Work out the finished part from the listing and answer in its coordinate system (mm). A direction names the side the tool comes from. Round coordinates to 2 decimals unless told otherwise and drop trailing zeros. Loops run counter-clockwise (first coordinate to the right, second up) from the corner with the lowest first, then second, coordinate; pieces in that order, holes last. Notation, with made-up numbers: (85, 84.25) - (101, 84.25) arc R24 cw to (101, 117.25) - close; hole circle Ø2 at (-37, 3.5). An arc over 180 degrees is marked (long way). Answer as CSV lines item,"result". Start each with the question number.
Q1. The mould has two halves that part along X. Classify faces 5 (the face through (1, 10, 10.16)), 6 (the face through (-10.39, 10.36, 6.26)), 7 (the face through (35, 8, 13.97)): +X half, -X half, draft (parallel to the pull), parting line (faces both ways), or undercut.
Q2. Straight lines are drawn through the part: L1, parallel to X at y = -0.75, z = 2; L2, parallel to X at y = 4.5, z = 10.25; L3, parallel to Y at x = -5.5, z = 12.5. For each, find the intervals that lie inside material, in ascending order. Write a range as [from, to].
Q3. Section D-D on z = 2.25 is taken. Count the separate pieces of the cut face and the enclosed holes in it, then the cut area to 3 significant figures.
Q4. Section A-A on y = -5 is taken. Write down the section's boundary in (x, z) (1 decimal), then the cut area to 3 significant figures.
Q5. For faces 1 (the face through (38.5, -7.43, 13.59)), 2 (the face through (20.7, 8.13, 13.61)), 3 (the face through (-5, -7, 10.16)), 4 (the face through (-7.97, 4.65, 13.61)), determine the directions among +Z, -Z, +X, -X, +Y, -Y from which every point of the face is accessible in a straight line to the end or side of a thin tool.
Q6. Section C-C on y = 2.25 is taken. Write down the section's boundary in (x, z) (1 decimal), then the cut area to 3 significant figures.
Q7. Section B-B on x = 26.5 is taken. Write down the section's boundary in (y, z).
Q8. Each of these flat-tipped pins is pushed along its axis until it touches: pin 1 Ø2 at (x, z) = (36.5, 11.5) entering from -Y; pin 2 Ø2 at (x, y) = (28, -7.5) entering from -Z; pin 3 Ø1.5 at (x, y) = (0, -11.5) entering from +Z; pin 4 Ø8 at (y, z) = (-9.5, 8) entering from -X. Where does it stop, or does it pass through?
```python
from build123d import *

# Parameters (mm, degrees)
F1_DEPTH        = 10.16
F2_DEPTH        = 13.97
F3_DEPTH        = 10.16
F8_R            = 5.08
F9_R            = 1.27
F11_D           = 4.445
F11_CSINK_D     = 8.89
F11_CSINK_ANGLE = 90


with BuildPart() as f1:
    # F0 (on Top) → F1 (new body)
    with BuildSketch(Plane.XY):
        with BuildLine():
            Line((-4.2164, 11.888180349), (-11.8364, 11.888180349))
            Line((-11.8364, 11.888180349), (-11.8364, 4.268180349))
            Line((-11.8364, 4.268180349), (-6.8157005053, 4.268180349))
            ThreePointArc((-6.8157005053, 4.268180349), (-5.6470856878, 5.6988660368), (-4.2164, 6.8674808543))
            Line((-4.2164, 6.8674808543), (-4.2164, 11.888180349))
        make_face()
        with BuildLine():
            Line((-4.2164, 4.268180349), (-4.2164, 6.8674808543))
            ThreePointArc((-4.2164, 6.8674808543), (-5.6470856878, 5.6988660368), (-6.8157005053, 4.268180349))
            Line((-6.8157005053, 4.268180349), (-4.2164, 4.268180349))
        make_face()
        with BuildLine():
            Line((13.5636, 11.888180349), (5.9436, 11.888180349))
            Line((5.9436, 11.888180349), (5.9436, 6.8674808543))
            ThreePointArc((5.9436, 6.8674808543), (7.3742856878, 5.6988660368), (8.5429005053, 4.268180349))
            Line((8.5429005053, 4.268180349), (13.5636, 4.268180349))
            Line((13.5636, 4.268180349), (13.5636, 11.888180349))
        make_face()
        with BuildLine():
            Line((13.5636, -13.511819651), (13.5636, -5.891819651))
            Line((13.5636, -5.891819651), (8.5429005053, -5.891819651))
            ThreePointArc((8.5429005053, -5.891819651), (7.3742856878, -7.3225053388), (5.9436, -8.4911201562))
            Line((5.9436, -8.4911201562), (5.9436, -13.511819651))
            Line((5.9436, -13.511819651), (13.5636, -13.511819651))
        make_face()
        with BuildLine():
            Line((-4.2164, -8.4911201562), (-4.2164, -13.511819651))
            Line((-4.2164, -13.511819651), (5.9436, -13.511819651))
            Line((5.9436, -13.511819651), (5.9436, -8.4911201562))
            ThreePointArc((5.9436, -8.4911201562), (0.8636, -10.019319651), (-4.2164, -8.4911201562))
        make_face()
        with BuildLine():
            Line((-6.8157005053, -5.891819651), (-11.8364, -5.891819651))
            Line((-11.8364, -5.891819651), (-11.8364, -13.511819651))
            Line((-11.8364, -13.511819651), (-4.2164, -13.511819651))
            Line((-4.2164, -13.511819651), (-4.2164, -8.4911201562))
            ThreePointArc((-4.2164, -8.4911201562), (-5.6470856878, -7.3225053388), (-6.8157005053, -5.891819651))
        make_face()
        with BuildLine():
            Line((-6.8157005053, 4.268180349), (-11.8364, 4.268180349))
            Line((-11.8364, 4.268180349), (-11.8364, -5.891819651))
            Line((-11.8364, -5.891819651), (-6.8157005053, -5.891819651))
            ThreePointArc((-6.8157005053, -5.891819651), (-8.3439, -0.811819651), (-6.8157005053, 4.268180349))
        make_face()
        with BuildLine():
            Line((13.5636, -5.891819651), (13.5636, 4.268180349))
            Line((13.5636, 4.268180349), (8.5429005053, 4.268180349))
            ThreePointArc((8.5429005053, 4.268180349), (9.6807768626, 1.8406223227), (10.0711, -0.811819651))
            ThreePointArc((10.0711, -0.811819651), (9.6807768626, -3.4642616247), (8.5429005053, -5.891819651))
            Line((8.5429005053, -5.891819651), (13.5636, -5.891819651))
        make_face()
        with BuildLine():
            Line((5.9436, 11.888180349), (-4.2164, 11.888180349))
            Line((-4.2164, 11.888180349), (-4.2164, 6.8674808543))
            ThreePointArc((-4.2164, 6.8674808543), (0.8636, 8.395680349), (5.9436, 6.8674808543))
            Line((5.9436, 6.8674808543), (5.9436, 11.888180349))
        make_face()
        with BuildLine():
            ThreePointArc((8.5429005053, 4.268180349), (7.3742856878, 5.6988660368), (5.9436, 6.8674808543))
            Line((5.9436, 6.8674808543), (5.9436, 4.268180349))
            Line((5.9436, 4.268180349), (8.5429005053, 4.268180349))
        make_face()
        with BuildLine():
            Line((5.9436, -5.891819651), (5.9436, -8.4911201562))
            ThreePointArc((5.9436, -8.4911201562), (7.3742856878, -7.3225053388), (8.5429005053, -5.891819651))
            Line((8.5429005053, -5.891819651), (5.9436, -5.891819651))
        make_face()
        with BuildLine():
            Line((-4.2164, -5.891819651), (-6.8157005053, -5.891819651))
            ThreePointArc((-6.8157005053, -5.891819651), (-5.6470856878, -7.3225053388), (-4.2164, -8.4911201562))
            Line((-4.2164, -8.4911201562), (-4.2164, -5.891819651))
        make_face()
    extrude(amount=F1_DEPTH)

    # F0 (on Top) → F2 (join)
    with BuildSketch(Plane.XY):
        with BuildLine():
            Line((-6.8157005053, -5.891819651), (-11.8364, -5.891819651))
            Line((-11.8364, -5.891819651), (-11.8364, -13.511819651))
            Line((-11.8364, -13.511819651), (-4.2164, -13.511819651))
            Line((-4.2164, -13.511819651), (-4.2164, -8.4911201562))
            ThreePointArc((-4.2164, -8.4911201562), (-5.6470856878, -7.3225053388), (-6.8157005053, -5.891819651))
        make_face()
        with BuildLine():
            Line((-4.2164, -5.891819651), (-6.8157005053, -5.891819651))
            ThreePointArc((-6.8157005053, -5.891819651), (-5.6470856878, -7.3225053388), (-4.2164, -8.4911201562))
            Line((-4.2164, -8.4911201562), (-4.2164, -5.891819651))
        make_face()
        with BuildLine():
            Line((13.5636, -13.511819651), (13.5636, -5.891819651))
            Line((13.5636, -5.891819651), (8.5429005053, -5.891819651))
            ThreePointArc((8.5429005053, -5.891819651), (7.3742856878, -7.3225053388), (5.9436, -8.4911201562))
            Line((5.9436, -8.4911201562), (5.9436, -13.511819651))
            Line((5.9436, -13.511819651), (13.5636, -13.511819651))
        make_face()
        with BuildLine():
            Line((5.9436, -5.891819651), (5.9436, -8.4911201562))
            ThreePointArc((5.9436, -8.4911201562), (7.3742856878, -7.3225053388), (8.5429005053, -5.891819651))
            Line((8.5429005053, -5.891819651), (5.9436, -5.891819651))
        make_face()
        with BuildLine():
            Line((13.5636, 11.888180349), (5.9436, 11.888180349))
            Line((5.9436, 11.888180349), (5.9436, 6.8674808543))
            ThreePointArc((5.9436, 6.8674808543), (7.3742856878, 5.6988660368), (8.5429005053, 4.268180349))
            Line((8.5429005053, 4.268180349), (13.5636, 4.268180349))
            Line((13.5636, 4.268180349), (13.5636, 11.888180349))
        make_face()
        with BuildLine():
            ThreePointArc((8.5429005053, 4.268180349), (7.3742856878, 5.6988660368), (5.9436, 6.8674808543))
            Line((5.9436, 6.8674808543), (5.9436, 4.268180349))
            Line((5.9436, 4.268180349), (8.5429005053, 4.268180349))
        make_face()
        with BuildLine():
            Line((-4.2164, 11.888180349), (-11.8364, 11.888180349))
            Line((-11.8364, 11.888180349), (-11.8364, 4.268180349))
            Line((-11.8364, 4.268180349), (-6.8157005053, 4.268180349))
            ThreePointArc((-6.8157005053, 4.268180349), (-5.6470856878, 5.6988660368), (-4.2164, 6.8674808543))
            Line((-4.2164, 6.8674808543), (-4.2164, 11.888180349))
        make_face()
        with BuildLine():
            Line((-4.2164, 4.268180349), (-4.2164, 6.8674808543))
            ThreePointArc((-4.2164, 6.8674808543), (-5.6470856878, 5.6988660368), (-6.8157005053, 4.268180349))
            Line((-6.8157005053, 4.268180349), (-4.2164, 4.268180349))
        make_face()
    extrude(amount=F2_DEPTH)

    # F0 (on Top) → F3 (cut)
    with BuildSketch(Plane.XY):
        with BuildLine():
            Line((-4.2164, 4.268180349), (-4.2164, 6.8674808543))
            ThreePointArc((-4.2164, 6.8674808543), (-5.6470856878, 5.6988660368), (-6.8157005053, 4.268180349))
            Line((-6.8157005053, 4.268180349), (-4.2164, 4.268180349))
        make_face()
        with BuildLine():
            Line((-4.2164, -5.891819651), (-6.8157005053, -5.891819651))
            ThreePointArc((-6.8157005053, -5.891819651), (-5.6470856878, -7.3225053388), (-4.2164, -8.4911201562))
            Line((-4.2164, -8.4911201562), (-4.2164, -5.891819651))
        make_face()
        with BuildLine():
            Line((5.9436, -5.891819651), (5.9436, -8.4911201562))
            ThreePointArc((5.9436, -8.4911201562), (7.3742856878, -7.3225053388), (8.5429005053, -5.891819651))
            Line((8.5429005053, -5.891819651), (5.9436, -5.891819651))
        make_face()
        with BuildLine():
            ThreePointArc((8.5429005053, 4.268180349), (7.3742856878, 5.6988660368), (5.9436, 6.8674808543))
            Line((5.9436, 6.8674808543), (5.9436, 4.268180349))
            Line((5.9436, 4.268180349), (8.5429005053, 4.268180349))
        make_face()
    extrude(amount=F3_DEPTH, mode=Mode.SUBTRACT)


with BuildPart() as f4_1:
    # F4: copy of F1
    add(f1.part.moved(Location((25.654, 0, 0))))


with BuildPart() as f6_1:
    # F6: copy of F1
    add(f1.part.moved(Location((25.2984, 0, 0))))


with BuildPart() as f1_1:
    add(f1.part)

    # F7: union F6_1
    add(f6_1.part)

    # F8
    f8_edges = [f1_1.edges().sort_by_distance(p)[0] for p in [
        (-11.8364, 11.88818, 6.985),
        (38.862, 11.88818, 6.985),
        (38.862, -13.51182, 6.985),
        (-11.8364, -13.51182, 6.985),
    ]]
    fillet(f8_edges, radius=F8_R)

    # F9
    f9_edges = [f1_1.edges().sort_by_distance(p)[0] for p in [
        (-10.348502, 10.400283, 13.97),
        (-4.2164, 8.07818, 13.97),
        (-8.0264, 4.26818, 13.97),
        (-8.0264, -5.89182, 13.97),
        (-4.2164, -9.70182, 13.97),
        (-10.348502, -12.023922, 13.97),
        (5.9436, -9.70182, 13.97),
        (9.7028, -5.89182, 13.97),
        (13.5128, -5.89182, 13.97),
        (9.7028, -13.51182, 13.97),
        (13.5128, -13.51182, 13.97),
        (32.512, -13.51182, 13.97),
        (21.082, -9.70182, 13.97),
        (13.5128, 11.88818, 13.97),
        (9.7028, 11.88818, 13.97),
        (17.3228, 11.88818, 13.97),
        (5.9436, 8.07818, 13.97),
        (21.082, 8.07818, 13.97),
        (13.5128, 4.26818, 13.97),
        (9.7028, 4.26818, 13.97),
        (31.242, 8.07818, 13.97),
        (35.052, 4.26818, 13.97),
        (35.052, -5.89182, 13.97),
        (31.242, -9.70182, 13.97),
        (37.374102, 10.400283, 13.97),
        (37.374102, -12.023922, 13.97),
    ]]
    fillet(f9_edges, radius=F9_R)

    # F11 (through all)
    with Locations(Plane.XZ.offset(13.511819651)):
        with Locations((13.5128, 5.7118628174)):
            CounterSinkHole(F11_D / 2, F11_CSINK_D / 2, counter_sink_angle=F11_CSINK_ANGLE)


solid = f1_1.part
```
Findings:
1,face 5,"undercut"
1,face 6,"-X half"
1,face 7,"draft"
2,L1,"x = [-11.84, -8.34], [10.07, 16.95], [35.37, 38.86]"
2,L2,"x = [-11.84, -4.22], [5.94, 21.08], [31.24, 38.86]"
2,L3,"y = [-13.51, -5.89], [4.27, 11.89]"
3,separate pieces,"1"
3,enclosed holes,"2"
3,area,"729 mm^2"
4,outline,"(-11.8, 0) - (-7.3, 0) - (-7.3, 10.2) - (-11.8, 10.2) - close; (9.1, 0) - (18, 0) - (18, 10.2) - (9.1, 10.2) - close; (34.4, 0) - (38.9, 0) - (38.9, 10.2) - (34.4, 10.2) - close; hole circle Ø4.4 at (13.5, 5.7)"
4,area,"166 mm^2"
5,face 1,"+Z, +X, +Y, -Y"
5,face 2,"+Z, +Y, -Y"
5,face 3,"-Z"
5,face 4,"+Z, +X, -X"
6,outline,"(-11.8, 0) - (-7.8, 0) - (-7.8, 10.2) - (-11.8, 10.2) - close; (9.5, 0) - (17.5, 0) - (17.5, 10.2) - (9.5, 10.2) - close; (34.8, 0) - (38.9, 0) - (38.9, 10.2) - (34.8, 10.2) - close; hole circle Ø4.4 at (13.5, 5.7)"
6,area,"147 mm^2"
7,outline,"(-13.51, 0) - (-10.01, 0) - (-10.01, 10.16) - (-13.51, 10.16) - close; (8.39, 0) - (11.89, 0) - (11.89, 10.16) - (8.39, 10.16) - close"
8,pin 1,"stops at y = -13.21"
8,pin 2,"passes through"
8,pin 3,"stops at z = 10.16"
8,pin 4,"stops at x = -11.84"
